Check sheet for the modelled part. Datum: model origin and axes. Units: mm. Face numbers are marked on the shaded views. A direction names the side the tool comes from. Round coordinates to 2 decimals unless told otherwise and drop trailing zeros. Order: outer loops, then holes, each group sorted by start corner. A loop starts at its lowest first (then second) coordinate and runs counter-clockwise, first axis right, second up.
from build123d import *

# Parameters (mm, degrees)
PAD_DEPTH = 10


with BuildPart() as part:
    # Sketch → Pad (new body)
    with BuildSketch(Plane.XY):
        with BuildLine():
            Line((0, 0), (54, 0))
            ThreePointArc((59, -5), (57.535534, -1.464466), (54, 0))
            Line((59, -5), (59, -18.017197))
            ThreePointArc((53.585664, -23), (57.385876, -21.696306), (59, -18.017197))
            ThreePointArc((53.585664, -23), (28.896907, -26.125735), (7.6, -39))
            ThreePointArc((7.6, -39), (5.342456, -27.337237), (-4, -20))
            ThreePointArc((-4, -20), (3.565231, -11.113046), (0, 0))
        make_face()
    extrude(amount=PAD_DEPTH)


solid = part.part
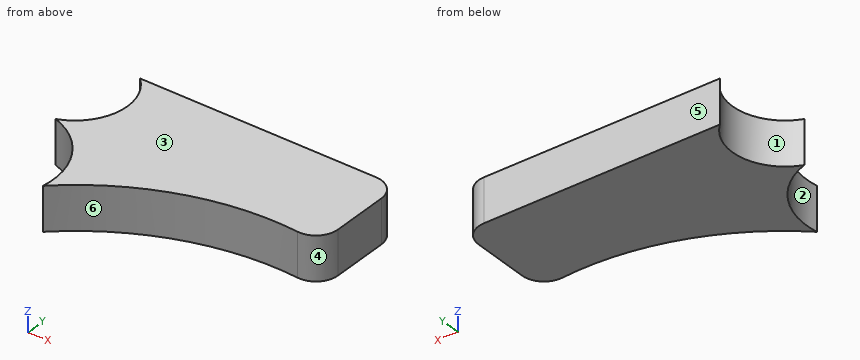
1) Sectioned sample at A-A on z = 6.5. Record the cut outline in (x, y).
2) Scan lines: line 1 (Y direction, x = 1, z = 9); line 2 (Y direction, x = 0.5, z = 9); line 3 (Y direction, x = 46, z = 4.5). Record each from-to range of solid material in increasing order.
3) Set-up check for the marked faces 5 and 6: record each of +Z, -Z, +X, -X, +Y, -Y from which the full face is reachable in a straight line by a thin tool's end or side.
4) Sectioned sample at B-B on y = -16. Record the cut outline in (x, z), and give its area (3 significant figures).
5) Draft check along Y on the marked faces 1, 2, 3 and 4. Enter one of: pulls with the +Y half, pulls with the -Y half, needs draft (parallel to the pull), parting line crosses it, or undercut.
6) Sectioned sample at C-C on x = 48. Record the cut outline in (y, z), and give its area (3 significant figures).
7) Gauge pin test, flat ends, axial feed: pin 1 (4 mm diameter, centred on x = 32, y = -25.5, fed in from -Z); pin 2 (5 mm diameter, centred on x = 43, z = 2.5, fed in from -Y); pin 3 (2 mm diameter, centred on x = 45.5, z = 2, fed in from -Y); pin 4 (4 mm diameter, centred on x = 30.5, z = 2.5, fed in from -Y). Record the tip position at first contact, or that the pin passes through.
Values found:
1. outline: (-4, -20) arc R17 cw to (7.6, -39) arc R60 cw to (53.59, -23) arc R5 ccw to (59, -18.02) - (59, -5) arc R5 ccw to (54, 0) - (0, 0) arc R12 cw to start
2. line 1: y = -22.57 to -16.46, -1.06 to 0
2. line 2: y = -22.21 to -17.02, -0.5 to 0
2. line 3: y = -22.85 to 0
3. face 5: +Z, -Z, +X, -X, +Y
3. face 6: +Z, -Z, -Y
4. outline: (1.37, 0) - (59, 0) - (59, 10) - (1.37, 10) - close
4. area: 576 mm2
5. face 1: undercut
5. face 2: undercut
5. face 3: needs draft
5. face 4: pulls with the -Y half
6. outline: (-22.8, 0) - (0, 0) - (0, 10) - (-22.8, 10) - close
6. area: 228 mm2
7. pin 1: stops at z = 0
7. pin 2: stops at y = -23.34
7. pin 3: stops at y = -22.93
7. pin 4: stops at y = -26.27
